Here's how the part is built. I have some questions about the finished solid (model axes, mm). A direction names the side the tool comes from. Coordinates: 2 decimals unless noted, no trailing zeros. Write each loop counter-clockwise with the first axis right and the second up, starting at its lowest first coordinate (ties: lowest second). Pieces come first, ordered by that corner, then holes. Notation, with made-up numbers: M 9,-0.5 L 50,-0.5 A26 cw 50,16.5 Z; hole C -7.5,89.25 d3. An arc over 180 degrees is marked long. Use one line per item in the form item = value. Start each with the question number.
1. I want a section at C-C, the plane y = 10.5. List the corners of the cut face in (x, z) for me.
2. Thinking about a two-plate mould opening in Y: for faces 4 (the face through (0, 47, -21)), 5 (the face through (36, -23, -16)), 6 (the face through (24.7, 52, -27.7)), 7 (the face through (40, 122, -10)), which applies, released by +Y, released by -Y, zero draft, split by the parting line, or undercut?
3. I want a section at B-B, the plane x = 37.5. List the corners of the cut face in (y, z) for me, plus the area to 3 significant figures.
4. On a 3-axis mill with a long thin cutter (end or side, diameter ignored), from which of +Z, -Z, +X, -X, +Y, -Y can I reach the whole of each face in a straight line? I mean faces 1 (the face through (40, 88, -30)), 2 (the face through (50, 122, -20)), 3 (the face through (39, -17, -14)). Say none if no direction works.
5. I want a section at A-A, the plane z = -9. List the corners of the cut face in (x, y) for me, plus the area to 3 significant figures.
6. I'm going to push flat-ended pins straight in: pin 1 Ø1 at (x, z) = (-21.5, -21.5) entering from -Y; pin 2 Ø11.5 at (x, z) = (-7.5, -8) entering from +Y; pin 3 Ø2 at (y, z) = (84, -22) entering from +X; pin 4 Ø3 at (y, z) = (113.3, -22.3) entering from -X. Where does each tip first touch, or does it pass through?
7. Please list where these lines run through material, in increasing order: line 1 along Y through (x, z) = (14, -22); line 2 along Z through (x, y) = (15, 113); line 3 along Y through (x, z) = (-0.5, -10). Write a range as [from, to].
8. I want a section at D-D, the plane y = -12.3. List the corners of the cut face in (x, z) for me.
from build123d import *

# Parameters (mm, degrees)
SKETCH_1_W           = 130
SKETCH_1_H           = 64
EXTRUDE_1_DEPTH      = 125
SKETCH_2_W           = 55.4
SKETCH_2_H           = 114
CUT_EXTRUDE_1_DEPTH  = 47
SKETCH_3_W           = 45.4
SKETCH_3_H           = 86
CUT_EXTRUDE_2_DEPTH  = 78
SKETCH_4_W           = 24.038907643
SKETCH_4_H           = 40
CUT_EXTRUDE_3_DEPTH  = 40
SKETCH_5_W           = 4.3
SKETCH_5_H           = 25
CUT_EXTRUDE_4_DEPTH  = 25
SKETCH_6_W           = 10
SKETCH_6_H           = 40
CUT_EXTRUDE_5_DEPTH  = 25
SKETCH_9_W           = 5
SKETCH_9_H           = 125
CUT_EXTRUDE_8_DEPTH  = 155.744951452
SKETCH_12_W          = 32
SKETCH_12_H          = 30
CUT_EXTRUDE_10_DEPTH = 155.744951452
SKETCH_13_W          = 45
SKETCH_13_H          = 64
CUT_EXTRUDE_11_DEPTH = 30
SKETCH_14_W          = 32
SKETCH_14_H          = 157.482614071
CUT_EXTRUDE_12_DEPTH = 180.649659059
SKETCH_18_W          = 30
SKETCH_18_H          = 95
CUT_EXTRUDE_15_DEPTH = 145.478372084
SKETCH_19_W          = 35
SKETCH_19_H          = 86
EXTRUDE_4_DEPTH      = 3
SKETCH_20_W          = 20
SKETCH_20_H          = 6
CUT_EXTRUDE_16_DEPTH = 150.244765402
FILLET_1_R           = 5
SKETCH_21_W          = 42
SKETCH_21_H          = 27.7
CUT_EXTRUDE_17_DEPTH = 138.927517197
EXTRUDE_7_DEPTH      = 27.7
SKETCH_23_W          = 48
SKETCH_23_H          = 4.3
EXTRUDE_8_DEPTH      = 23
SKETCH_25_R          = 1.55
CUT_EXTRUDE_19_DEPTH = 138.669895039
FILLET_3_R           = 5


with BuildPart() as part:
    # 草图1 → 凸台-拉伸1 (new body)
    with BuildSketch(Plane(origin=(0, 0, 0), x_dir=(1, 0, 0), z_dir=(0, 1, 0))):
        Rectangle(SKETCH_1_W, SKETCH_1_H)
    extrude(amount=EXTRUDE_1_DEPTH)

    # 草图2 → 切除-拉伸1 (cut)
    with BuildSketch(Plane(origin=(65, 0, 0), x_dir=(0, 0, -1), z_dir=(1, 0, 0))):
        with Locations((0, 62)):
            Rectangle(SKETCH_2_W, SKETCH_2_H)
    extrude(amount=-CUT_EXTRUDE_1_DEPTH, mode=Mode.SUBTRACT)

    # 草图3 → 切除-拉伸2 (cut)
    with BuildSketch(Plane(origin=(18, 0, 0), x_dir=(0, 0, -1), z_dir=(1, 0, 0))):
        with Locations((0, 48)):
            Rectangle(SKETCH_3_W, SKETCH_3_H)
    extrude(amount=-CUT_EXTRUDE_2_DEPTH, mode=Mode.SUBTRACT)

    # 草图4 → 切除-拉伸3 (cut)
    with BuildSketch(Plane(origin=(65, 0, 0), x_dir=(0, 0, -1), z_dir=(1, 0, 0))):
        with Locations((26.569318974, 55)):
            Rectangle(SKETCH_4_W, SKETCH_4_H)
    extrude(amount=-CUT_EXTRUDE_3_DEPTH, mode=Mode.SUBTRACT)

    # 草图5 → 切除-拉伸4 (cut)
    with BuildSketch(Plane(origin=(65, 0, 0), x_dir=(0, 0, -1), z_dir=(1, 0, 0))):
        with Locations((29.85, 87.5)):
            Rectangle(SKETCH_5_W, SKETCH_5_H)
    extrude(amount=-CUT_EXTRUDE_4_DEPTH, mode=Mode.SUBTRACT)

    # 草图6 → 切除-拉伸5 (cut)
    with BuildSketch(Plane(origin=(0, 125, 0), x_dir=(1, 0, 0), z_dir=(0, 1, 0))):
        with Locations((45, 0)):
            Rectangle(SKETCH_6_W, SKETCH_6_H)
    extrude(amount=-CUT_EXTRUDE_5_DEPTH, mode=Mode.SUBTRACT)

    # 草图9 → 切除-拉伸8 (cut, through all)
    with BuildSketch(Plane.XY.offset(32)):
        with Locations((62.5, 62.5)):
            Rectangle(SKETCH_9_W, SKETCH_9_H)
    extrude(amount=-CUT_EXTRUDE_8_DEPTH, mode=Mode.SUBTRACT)

    # 草图12 → 切除-拉伸10 (cut, through all)
    with BuildSketch(Plane.XY.offset(32)):
        with Locations((-49, 110)):
            Rectangle(SKETCH_12_W, SKETCH_12_H)
    extrude(amount=-CUT_EXTRUDE_10_DEPTH, mode=Mode.SUBTRACT)

    # 草图13 → 切除-拉伸11 (cut)
    with BuildSketch(Plane(origin=(0, 125, 0), x_dir=(1, 0, 0), z_dir=(0, 1, 0))):
        with Locations((-10.5, 0)):
            Rectangle(SKETCH_13_W, SKETCH_13_H)
    extrude(amount=-CUT_EXTRUDE_11_DEPTH, mode=Mode.SUBTRACT)

    # 草图14 → 切除-拉伸12 (cut, through all)
    with BuildSketch(Plane.ZY.offset(65)):
        with Locations((16, 78.741307036)):
            Rectangle(SKETCH_14_W, SKETCH_14_H)
    extrude(amount=-CUT_EXTRUDE_12_DEPTH, mode=Mode.SUBTRACT)

    # 草图18 → 切除-拉伸15 (cut, through all)
    with BuildSketch(Plane.XY):
        with Locations((-50, 47.5)):
            Rectangle(SKETCH_18_W, SKETCH_18_H)
    extrude(amount=-CUT_EXTRUDE_15_DEPTH, mode=Mode.SUBTRACT)

    # 草图19 → 凸台-拉伸4 (add)
    with BuildSketch(Plane.XY.offset(-22.7)):
        with Locations((-17.5, 48)):
            Rectangle(SKETCH_19_W, SKETCH_19_H)
    extrude(amount=EXTRUDE_4_DEPTH)

    # 草图20 → 切除-拉伸16 (cut, through all)
    with BuildSketch(Plane(origin=(40, 0, 0), x_dir=(0, 0, -1), z_dir=(1, 0, 0))):
        with Locations((10, 122)):
            Rectangle(SKETCH_20_W, SKETCH_20_H)
    extrude(amount=CUT_EXTRUDE_16_DEPTH, mode=Mode.SUBTRACT)

    # 圆角1
    fillet_1_edges = [part.edges().sort_by_distance(p)[0] for p in [
        (12, 95, -16),
    ]]
    fillet(fillet_1_edges, radius=FILLET_1_R)

    # 草图21 → 切除-拉伸17 (cut, through all)
    with BuildSketch(Plane(origin=(0, 5, 0), x_dir=(1, 0, 0), z_dir=(0, 1, 0))):
        with Locations((39, 13.85)):
            Rectangle(SKETCH_21_W, SKETCH_21_H)
    extrude(amount=-CUT_EXTRUDE_17_DEPTH, mode=Mode.SUBTRACT)

    # 草图22 → 凸台-拉伸7 (add)
    with BuildSketch(Plane.XY):
        Polygon((12, 0), (18, 0), (18, -17), (60, -17), (60, -23), (12, -23), align=None)
    extrude(amount=-EXTRUDE_7_DEPTH)

    # 草图23 → 凸台-拉伸8 (add)
    with BuildSketch(Plane.XZ):
        with Locations((36, -29.85)):
            Rectangle(SKETCH_23_W, SKETCH_23_H)
    extrude(amount=EXTRUDE_8_DEPTH)

    # 草图25 → 切除-拉伸19 (cut, through all)
    with BuildSketch(Plane.ZY.offset(-12)):
        with Locations(Location((-22.3, 113.3, 0), (0, 0, 270))):
            Circle(SKETCH_25_R)
        with Locations(Location((-22.3, -12.3, 0), (0, 0, 270))):
            Circle(SKETCH_25_R)
    extrude(amount=-CUT_EXTRUDE_19_DEPTH, mode=Mode.SUBTRACT)

    # 圆角3
    fillet_3_edges = [part.edges().sort_by_distance(p)[0] for p in [
        (12, 0, -16),
    ]]
    fillet(fillet_3_edges, radius=FILLET_3_R)


solid = part.part
Answer list:
q1.outline = M -35,-32 L 60,-32 L 60,-27.7 L 18,-27.7 L 18,-22.7 L 0,-22.7 L 0,-19.7 L -35,-19.7 Z
q2.face_4 = undercut
q2.face_5 = released by -Y
q2.face_6 = undercut
q2.face_7 = zero draft
q3.outline = M -23,-32 L 35,-32 L 35,-27.7 L -17,-27.7 L -17,0 L -23,0 Z; M 75,-32 L 125,-32 L 125,0 L 119,0 L 119,-27.7 L 75,-27.7 Z
q3.area = 797 mm²
q4.face_1 = +Z, -Z, +X
q4.face_2 = +Z, +X, +Y
q4.face_3 = +Z, +X
q5.outline = M -35,0 L 7,0 A5 cw 12,-5 L 12,-23 L 60,-23 L 60,-17 L 18,-17 L 18,5 L -35,5 Z; M -35,91 L 18,91 L 18,119 L 40,119 L 40,125 L 12,125 L 12,100 A5 cw 7,95 L -35,95 Z
q5.area = 1,190 mm²
q6.pin_1 = 0
q6.pin_2 = 95
q6.pin_3 = 18
q6.pin_4 = through
q7.line_1 = [-23, -13.82], [-10.78, 5], [91, 111.78], [114.82, 125]
q7.line_2 = [-32, -23.82], [-20.78, 0]
q7.line_3 = [0, 5], [91, 95]
q8.outline = M 12,-32 L 60,-32 L 60,-27.7 L 18,-27.7 L 18,-23.85 L 12,-23.85 Z; M 12,-20.75 L 18,-20.75 L 18,0 L 12,0 Z
